Check sheet for the modelled part. Datum: model origin and axes. Units: mm. A direction names the side the tool comes from. Coordinates: 2 decimals unless noted, no trailing zeros. Write each loop counter-clockwise with the first axis right and the second up, starting at its lowest first coordinate (ties: lowest second). Pieces come first, ordered by that corner, then holes. Notation, with made-up numbers: (77.5, 72) - (128.5, 72) arc R18 cw to (128.5, 82) - close; hole circle Ø8 at (87.5, 31.25). An arc over 180 degrees is marked (long way). Answer as CSV lines item,"result". Start each with the question number.
from build123d import *

# Parameters (mm, degrees)
SKETCH1_W           = 80
SKETCH1_H           = 80
BOSS_EXTRUDE1_DEPTH = 35
CUT_EXTRUDE1_REACH  = 120.427
CUT_EXTRUDE2_DEPTH  = 35


with BuildPart() as part:
    # Sketch1 → Boss-Extrude1 (new body)
    with BuildSketch(Plane.XY):
        with Locations((-40, 40)):
            Rectangle(SKETCH1_W, SKETCH1_H)
    extrude(amount=BOSS_EXTRUDE1_DEPTH)

    # Sketch4 → Cut-Extrude1 (cut, up to next)
    with BuildSketch(Plane.XZ, mode=Mode.PRIVATE) as cut_extrude1_sk1:
        Polygon((-80, 35), (0, 15), (0, 35), align=None)
    cut_extrude1_tool1 = extrude(cut_extrude1_sk1.sketch, amount=-CUT_EXTRUDE1_REACH, mode=Mode.PRIVATE) & part.part
    add(cut_extrude1_tool1.solids().sort_by_distance((-26.666667, 0, 28.333333))[0], mode=Mode.SUBTRACT)

    # Sketch5 → Cut-Extrude2 (cut)
    with BuildSketch(Plane(origin=(0, 0, 0), x_dir=(-1, 0, 0), z_dir=(0, 0, -1))):
        with BuildLine():
            Line((34, 69.393876913), (34, 64.269322199))
            ThreePointArc((34, 64.269322199), (22.32233047, 57.67766953), (15.730677801, 46))
            Line((15.730677801, 46), (10.606123087, 46))
            ThreePointArc((10.606123087, 46), (10, 40), (10.606123087, 34))
            Line((10.606123087, 34), (15.730677801, 34))
            ThreePointArc((15.730677801, 34), (22.32233047, 22.32233047), (34, 15.730677801))
            Line((34, 15.730677801), (34, 10.606123087))
            ThreePointArc((34, 10.606123087), (40, 10), (46, 10.606123087))
            Line((46, 10.606123087), (46, 15.730677801))
            ThreePointArc((46, 15.730677801), (57.67766953, 22.32233047), (64.269322199, 34))
            Line((64.269322199, 34), (69.393876913, 34))
            ThreePointArc((69.393876913, 34), (70, 40), (69.393876913, 46))
            Line((69.393876913, 46), (64.269322199, 46))
            ThreePointArc((64.269322199, 46), (57.67766953, 57.67766953), (46, 64.269322199))
            Line((46, 64.269322199), (46, 69.393876913))
            ThreePointArc((46, 69.393876913), (40, 70), (34, 69.393876913))
        make_face()
        Polygon((5.358983849, 60), (40, 80), (0, 80), (0, 0), (40, 0), (5.358983849, 20), align=None)
        Polygon((80, 80), (40, 80), (74.641016151, 60), (74.641016151, 20), (40, 0), (80, 0), align=None)
    extrude(amount=-CUT_EXTRUDE2_DEPTH, mode=Mode.SUBTRACT)


solid = part.part
(1) Cross-section at D-D on z = 30. Record the boundary of the cut face in (x, y), plus the area to 3 significant figures.
(2) Tool access check on faces 4 (the face through (-74.641, 40, 17)), 5 (the face through (-46, 67, 13)). Record the directions out of +Z, -Z, +X, -X, +Y, -Y that give a thin tool (end or side, any length) a straight path to the whole face; none if there is none.
(3) Material ranges on probe 1 along Y at (x, z) = (-37, 8.5); probe 2 along Y at (x, z) = (-49, 24); probe 3 along X at (y, z) = (15, 13), recorded low to high. Write a range as from..to.
(4) Go/stop test with flat-tipped pins: P1, Ø4, axis at y = 13, z = 11.5, coming from the -X side; P2, Ø5.5, axis at x = -67.5, z = 20.5, coming from the -Y side; P3, Ø12, axis at x = -38.5, y = 57.5, coming from the +Z side; P4, Ø1.5, axis at x = -14.5, z = 9, coming from the +Y side. Record where each tip stops, or that it passes through.
(5) Cross-section at A-A on z = 10. Record the boundary of the cut face in (x, y).
(6) Cross-section at C-C on x = -44. Record the boundary of the cut face in (y, z), plus the area to 3 significant figures.
(7) Cross-section at B-B on y = 62. Record the boundary of the cut face in (x, z).
(8) Release check for a two-part mould opening along X. For faces 1 (the face through (-64, 48, 31)), 2 (the face through (-57.56, 10.14, 12.85)), 3 (the face through (-10, 40, 9)) record: pulls with the +X half, pulls with the -X half, needs draft (parallel to the pull), parting line crosses it, or undercut.
Checked values:
1,outline,"(-74.64, 20) - (-60, 11.55) - (-60, 25) arc R25 cw to (-64.27, 34) - (-69.39, 34) arc R30 cw to (-69.39, 46) - (-64.27, 46) arc R25 cw to (-60, 55) - (-60, 68.45) - (-74.64, 60) - close"
1,area,"547 mm^2"
2,face 4,"+Z, -Z, -X, +Y, -Y"
2,face 5,"+Z, -Z"
3,probe 1,"1.73..10.15, 69.85..78.27"
3,probe 2,"5.2..16.68, 63.32..74.8"
3,probe 3,"-65.98..-46, -34..-14.02"
4,P1,"x = -65.98"
4,P2,"y = 14.29"
4,P3,"through"
4,P4,"y = 65.71"
5,outline,"(-74.64, 20) - (-40, 0) - (-5.36, 20) - (-5.36, 60) - (-40, 80) - (-74.64, 60) - close; hole (-69.39, 34) - (-64.27, 34) arc R25 ccw to (-46, 15.73) - (-46, 10.61) arc R30 ccw to (-34, 10.61) - (-34, 15.73) arc R25 ccw to (-15.73, 34) - (-10.61, 34) arc R30 ccw to (-10.61, 46) - (-15.73, 46) arc R25 ccw to (-34, 64.27) - (-34, 69.39) arc R30 ccw to (-46, 69.39) - (-46, 64.27) arc R25 ccw to (-64.27, 46) - (-69.39, 46) arc R30 ccw to start"
6,outline,"(2.31, 0) - (10.27, 0) - (10.27, 26) - (2.31, 26) - close; (69.73, 0) - (77.69, 0) - (77.69, 26) - (69.73, 26) - close"
6,area,"414 mm^2"
7,outline,"(-71.18, 0) - (-51.87, 0) - (-51.87, 27.97) - (-71.18, 32.79) - close; (-28.13, 0) - (-8.82, 0) - (-8.82, 17.21) - (-28.13, 22.03) - close"
8,face 1,"pulls with the +X half"
8,face 2,"pulls with the -X half"
8,face 3,"undercut"
